Can you work these out from the model? Positions are in its coordinate system, mm. A direction names the side the tool comes from. Give positions to 0.01 mm unless a question says otherwise; leave off trailing zeros. Order: outer loops, then holes, each group sorted by start corner. A loop starts at its lowest first (then second) coordinate and runs counter-clockwise, first axis right, second up. Notation, with made-up numbers: (10.25, 16.5) - (52.25, 16.5) arc R21 cw to (52.25, 48.5) - close; hole circle Ø7 at (61.5, 75). An arc over 180 degrees is marked (long way). Answer as a JSON object with one key per item and string values.
```python
from build123d import *

# Parameters (mm, degrees)
BOSS_EXTRUDE1_DEPTH = 2
BOSS_EXTRUDE2_DEPTH = 103
BOSS_EXTRUDE3_DEPTH = 2
SKETCH4_W           = 103
SKETCH4_H           = 43
CUT_EXTRUDE1_DEPTH  = 2
SKETCH5_W           = 91
SKETCH5_H           = 5
CUT_EXTRUDE2_DEPTH  = 0.5
SKETCH7_W           = 105
SKETCH7_H           = 85.5
SKETCH7_W_2         = 103
SKETCH7_H_2         = 83.5
CUT_EXTRUDE3_DEPTH  = 1.5
CUT_EXTRUDE4_REACH  = 142.164
SKETCH8_W           = 91
SKETCH8_H           = 11
CUT_EXTRUDE5_REACH  = 119.914
SKETCH9_W           = 6
SKETCH9_H           = 2.5
FILLET1_R           = 1


with BuildPart() as part:
    # Sketch1 → Boss-Extrude1 (new body)
    with BuildSketch(Plane(origin=(0, 0, 0), x_dir=(0, 0, -1), z_dir=(1, 0, 0))):
        Polygon((-43.75, -23.25), (43.75, -23.25), (43.75, -6.25), (31, -6.25), (31, 12.75), (23.5, 12.75), (23.5, 23.25), (-23.5, 23.25), (-23.5, 12.75), (-31, 12.75), (-31, -6.25), (-43.75, -6.25), align=None)
    extrude(amount=-BOSS_EXTRUDE1_DEPTH)

    # Sketch2 → Boss-Extrude2 (add)
    with BuildSketch(Plane.ZY.offset(2)):
        Polygon((-43.75, -23.25), (-43.75, -6.25), (-31, -6.25), (-31, 12.75), (-23.5, 12.75), (-23.5, 23.25), (23.5, 23.25), (23.5, 12.75), (31, 12.75), (31, -6.25), (43.75, -6.25), (43.75, -23.25), (41.75, -23.25), (41.75, -7.25), (28.5, -7.25), (28.5, 11.75), (22.5, 11.75), (22.5, 19.75), (-22.5, 19.75), (-22.5, 11.75), (-28.5, 11.75), (-28.5, -7.25), (-41.75, -7.25), (-41.75, -23.25), align=None)
    extrude(amount=BOSS_EXTRUDE2_DEPTH)

    # Sketch3 → Boss-Extrude3 (add)
    with BuildSketch(Plane.ZY.offset(105)):
        Polygon((43.75, -23.25), (43.75, -6.25), (31, -6.25), (31, 12.75), (23.5, 12.75), (23.5, 23.25), (-23.5, 23.25), (-23.5, 12.75), (-31, 12.75), (-31, -6.25), (-43.75, -6.25), (-43.75, -23.25), align=None)
    extrude(amount=BOSS_EXTRUDE3_DEPTH)

    # Sketch4 → Cut-Extrude1 (cut)
    with BuildSketch(Plane(origin=(0, 23.25, 0), x_dir=(1, 0, 0), z_dir=(0, 1, 0))):
        with Locations((-53.5, 0)):
            Rectangle(SKETCH4_W, SKETCH4_H)
    extrude(amount=-CUT_EXTRUDE1_DEPTH, mode=Mode.SUBTRACT)

    # Sketch5 → Cut-Extrude2 (cut)
    with BuildSketch(Plane(origin=(0, -6.25, 0), x_dir=(1, 0, 0), z_dir=(0, 1, 0))):
        with Locations((-53.5, -38.75)):
            Rectangle(SKETCH5_W, SKETCH5_H)
        with Locations((-53.5, 38.75)):
            Rectangle(SKETCH5_W, SKETCH5_H)
    extrude(amount=-CUT_EXTRUDE2_DEPTH, mode=Mode.SUBTRACT)

    # Sketch7 → Cut-Extrude3 (cut)
    with BuildSketch(Plane.XZ.offset(23.25)):
        with Locations((-53.5, 0)):
            Rectangle(SKETCH7_W, SKETCH7_H)
        with Locations((-53.5, 0)):
            Rectangle(SKETCH7_W_2, SKETCH7_H_2, mode=Mode.SUBTRACT)
    extrude(amount=-CUT_EXTRUDE3_DEPTH, mode=Mode.SUBTRACT)

    # Cut-Extrude4: up to this face of the body (flat: up to its plane)
    cut_extrude4_end = Plane(part.part.faces().sort_by_distance((-53.5, -14.75, -43.75))[0])
    # Sketch8 → Cut-Extrude4 (cut, up to the picked face)
    with BuildSketch(Plane.XY.offset(43.75), mode=Mode.PRIVATE) as cut_extrude4_sk1:
        with Locations((-53.5, -17.75)):
            Rectangle(SKETCH8_W, SKETCH8_H)
    cut_extrude4_tool1 = split(extrude(cut_extrude4_sk1.sketch, amount=-CUT_EXTRUDE4_REACH, mode=Mode.PRIVATE), bisect_by=cut_extrude4_end, keep=Keep.BOTH, mode=Mode.PRIVATE)
    add(cut_extrude4_tool1.solids().sort_by(Axis((-53.5, -17.75, 43.75), (0, 0, -1)))[0], mode=Mode.SUBTRACT)

    # Cut-Extrude5: up to this face of the body (flat: up to its plane)
    cut_extrude5_end = Plane(part.part.faces().sort_by_distance((-107, -2.921533713, 0))[0])
    # Sketch9 → Cut-Extrude5 (cut, up to the picked face)
    with BuildSketch(Plane(origin=(0, 0, 0), x_dir=(0, 0, -1), z_dir=(1, 0, 0)), mode=Mode.PRIVATE) as cut_extrude5_sk1:
        with Locations((0, -17.5)):
            Rectangle(SKETCH9_W, SKETCH9_H)
    cut_extrude5_tool1 = split(extrude(cut_extrude5_sk1.sketch, amount=-CUT_EXTRUDE5_REACH, mode=Mode.PRIVATE), bisect_by=cut_extrude5_end, keep=Keep.BOTH, mode=Mode.PRIVATE)
    add(cut_extrude5_tool1.solids().sort_by(Axis((0, -17.5, 0), (-1, 0, 0)))[0], mode=Mode.SUBTRACT)

    # Fillet1
    fillet1_edges = [part.edges().sort_by_distance(p)[0] for p in [
        (-107, -6.25, 37.375),
        (-107, 3.25, 31),
        (-107, 12.75, 27.25),
        (-107, 18, 23.5),
        (-107, 23.25, 0),
        (-107, 18, -23.5),
        (-107, 12.75, -27.25),
        (-107, 3.25, -31),
        (-107, -6.25, -37.375),
        (-107, -14.75, -43.75),
        (-107, -14.75, 43.75),
        (0, -6.25, 37.375),
        (0, 3.25, 31),
        (0, 12.75, 27.25),
        (0, 18, 23.5),
        (0, 23.25, 0),
        (0, 18, -23.5),
        (0, 12.75, -27.25),
        (0, 3.25, -31),
        (0, -6.25, -37.375),
        (0, -14.75, -43.75),
        (0, -14.75, 43.75),
        (-53.5, -6.25, 43.75),
        (-53.5, 12.75, 31),
        (-53.5, 23.25, 23.5),
        (-53.5, 23.25, -23.5),
        (-53.5, 12.75, -31),
        (-53.5, -6.25, -43.75),
    ]]
    fillet(fillet1_edges, radius=FILLET1_R)


solid = part.part
```
Q1. If we section it at D-D, the plane z = -7.5: Please give me the cut outline in (x, y), then the cut area to 3 significant figures.
Recorded:
{"outline": "(-107, -23.25) - (-106, -23.25) - (-106, -21.75) - (-105, -21.75) - (-105, 19.75) - (-2, 19.75) - (-2, -21.75) - (-1, -21.75) - (-1, -23.25) - (0, -23.25) - (0, 22.25) arc R1 ccw to (-1, 23.25) - (-2, 23.25) - (-2, 21.25) - (-105, 21.25) - (-105, 23.25) - (-106, 23.25) arc R1 ccw to (-107, 22.25) - close", "area": "337 mm^2"}
Q2. Which directions (+Z, -Z, +X, -X, +Y, -Y) give clear straight access to the entire face, cutting with the end or side of a thin tool? Please do faces 4 (the face through (-53, 3, 31)), 5 (the face through (-105.6, -21.75, 0.2)), 6 (the face through (-54, 21.25, 0)).
Recorded:
{"face 4": "+Z, +X, -X, +Y", "face 5": "-Y", "face 6": "+Y"}
Q3. I need wall thicknesses on L1, parallel to Z at x = -59, y = -8; L2, parallel to Z at x = -75.5, y = -4.5; L3, parallel to X at y = 9.5, z = 26.5. Which ranges of each line are inside material? Lowest first, please.
Recorded:
{"L1": "z = -43.75 to -41.75, 41.75 to 43.75", "L2": "z = -31 to -28.5, 28.5 to 31", "L3": "x = -107 to -105, -2 to 0"}
Q4. If we section it at B-B, the plane z = 25.5: Please give me the cut outline in (x, y), then the cut area to 3 significant figures.
Recorded:
{"outline": "(-107, -23.25) - (-106, -23.25) - (-106, -21.75) - (-105, -21.75) - (-105, 11.75) - (-2, 11.75) - (-2, -21.75) - (-1, -21.75) - (-1, -23.25) - (0, -23.25) - (0, 11.75) arc R1 ccw to (-1, 12.75) - (-106, 12.75) arc R1 ccw to (-107, 11.75) - close", "area": "244 mm^2"}
Q5. If we section it at C-C, the plane y = 17.5: Please give me the cut outline in (x, z), then the cut area to 3 significant figures.
Recorded:
{"outline": "(-107, -22.5) arc R1 ccw to (-106, -23.5) - (-1, -23.5) arc R1 ccw to (0, -22.5) - (0, 22.5) arc R1 ccw to (-1, 23.5) - (-106, 23.5) arc R1 ccw to (-107, 22.5) - close; hole (-105, -22.5) - (-2, -22.5) - (-2, 22.5) - (-105, 22.5) - close", "area": "393 mm^2"}
Q6. I'm going to push flat-ended pins straight in: pin 1 Ø3.5 at (x, z) = (-5, 1) entering from -Y; pin 2 Ø4 at (x, y) = (-75.5, 0.5) entering from +Z; pin 3 Ø5.5 at (x, z) = (-103, 13) entering from -Y; pin 4 Ø6 at (x, y) = (-33.5, -17) entering from -Z. Where does each tip first touch, or does it pass through?
Recorded:
{"pin 1": "stops at y = 19.75", "pin 2": "stops at z = 31", "pin 3": "stops at y = -21.75", "pin 4": "passes through"}
Q7. If we section it at A-A, the plane y = -4.5: Please give me the cut outline in (x, z).
Recorded:
{"outline": "(-107, -30) arc R1 ccw to (-106, -31) - (-1, -31) arc R1 ccw to (0, -30) - (0, 30) arc R1 ccw to (-1, 31) - (-106, 31) arc R1 ccw to (-107, 30) - close; hole (-105, -28.5) - (-2, -28.5) - (-2, 28.5) - (-105, 28.5) - close"}
Q8. We'd pull the mould along Z, two halves only. Please class faces 1 (the face through (-53, 17, 23.5)), 2 (the face through (-53, -6.25, 36)), 3 (the face through (-53, 19.75, 0)): released by +Z, released by -Z, zero draft, split by the parting line, or undercut.
Recorded:
{"face 1": "released by +Z", "face 2": "zero draft", "face 3": "undercut"}
